from build123d import *

# Parameters (mm, degrees)
F0_W     = 136.9934380054
F0_H     = 98.2272103429
F1_DEPTH = 125
F2_DEPTH = 108
F3_T     = -2.5


with BuildPart() as f1:
    # F0 (on Front) → F1 (new body)
    with BuildSketch(Plane.XZ):
        Rectangle(F0_W, F0_H)
    extrude(amount=F1_DEPTH)

    # F2 (add): a face of the model
    f2_faces = [f1.faces().sort_by_distance(p)[0] for p in [
        (0, -62.5, 49.1136051714),
    ]]
    extrude(f2_faces, amount=F2_DEPTH)

    # F3
    f3_openings = [f1.faces().sort_by_distance(p)[0] for p in [
        (0, -62.5, 157.113605),
    ]]
    offset(amount=F3_T, openings=f3_openings)


solid = f1.part
For this review, take the finished solid that the model builds, in its own axes (mm). A direction names the side the tool comes from. Give positions to 0.01 mm unless a question says otherwise; leave off trailing zeros. Order: outer loops, then holes, each group sorted by start corner. A loop starts at its lowest first (then second) coordinate and runs counter-clockwise, first axis right, second up. Notation, with made-up numbers: M -31,16 L -9,16 A10 cw -9,22 Z; hole C 37.25,46.25 d9. An arc over 180 degrees is marked long. Answer in a Markdown table with one row per item. Add a question column.
(1) Consider section A-A on z = -10. State the section outline as (x, y) points, and give its area (3 significant figures).
(2) For faces 5 (the face through (-1, -62, -46.614)), 6 (the face through (-1, -62, -49.114)), list the 3-axis set-ups (+Z, -Z, +X, -X, +Y, -Y) from which the entire face can be reached by the end or side of a thin tool; tool diameter is ignored.
(3) Wall thickness on probe 1 along X at (y, z) = (-104.5, 50); probe 2 along Y at (x, z) = (-9.5, 146.5); probe 3 along Z at (x, y) = (43, -57): over which ranges is each line inside the solid? List them lowest first. Write a range as [from, to].
(4) Consider section B-B on y = -48.5. State the section outline as (x, z) points.
(5) Mouldability with a two-part tool opening along Y and no side actions: class faces 1 (the face through (-1, -125, 53)), 2 (the face through (65.997, -62, 54)), 3 (the face through (-31, -2, 157.114)), 4 (the face through (-65.997, -62, 54)) as +Y half, -Y half, draft (parallel to the pull), parting line (faces both ways), or undercut.
(6) For pin 1 (10 mm diameter, centred on x = 4, y = -44, fed in from +Z), flat-tipped, find the tip position at first contact; note if it passes through.
(7) Consider section C-C on x = 28. State the section outline as (y, z) points, and give its area (3 significant figures).
Evaluation:
| question | item | result |
|---|---|---|
| 1 | outline | M -68.5,-125 L 68.5,-125 L 68.5,0 L -68.5,0 Z; hole M -66,-122.5 L 66,-122.5 L 66,-2.5 L -66,-2.5 Z |
| 1 | area | 1,280 mm^2 |
| 2 | face 5 | +Z |
| 2 | face 6 | -Z, +X, -X, +Y, -Y |
| 3 | probe 1 | x = [-68.5, -66], [66, 68.5] |
| 3 | probe 2 | y = [-125, -122.5], [-2.5, 0] |
| 3 | probe 3 | z = [-49.11, -46.61] |
| 4 | outline | M -68.5,-49.11 L 68.5,-49.11 L 68.5,157.11 L 66,157.11 L 66,-46.61 L -66,-46.61 L -66,157.11 L -68.5,157.11 Z |
| 5 | face 1 | -Y half |
| 5 | face 2 | undercut |
| 5 | face 3 | draft |
| 5 | face 4 | undercut |
| 6 | pin 1 | stops at z = -46.61 |
| 7 | outline | M -125,-49.11 L 0,-49.11 L 0,157.11 L -2.5,157.11 L -2.5,-46.61 L -122.5,-46.61 L -122.5,157.11 L -125,157.11 Z |
| 7 | area | 1,330 mm^2 |
